Model file for the job. Use its own axes, mm. A direction names the side the tool comes from. Give positions to 0.01 mm unless a question says otherwise; leave off trailing zeros. Loops run counter-clockwise (first coordinate to the right, second up) from the corner with the lowest first, then second, coordinate; pieces in that order, holes last. Notation, with made-up numbers: M -1,-22 L 31,-22 A17 cw 31,0 Z; hole C -36.75,-20 d7. An arc over 180 degrees is marked long. Answer in a Markdown table with one row per item.
```python
from build123d import *

# Parameters (mm, degrees)
SKETCH1_W                 = 71.11
SKETCH1_H                 = 53.65
SKETCH1_R                 = 6.35
SKETCH1_R_2               = 1.5
BOSS_EXTRUDE1_DEPTH       = 6.35
F_8_CLEARANCE_HOLE1_D     = 4.4958
F_6_32_TAPPED_HOLE1_D     = 2.7051
F_6_32_TAPPED_HOLE1_DEPTH = 25.4
F_6_32_TAPPED_HOLE1_TIP   = 0.81269403
CUT_EXTRUDE1_DEPTH        = 7.35
FILLET1_R                 = 3.175


with BuildPart() as part:
    # Sketch1 → Boss-Extrude1 (new body)
    with BuildSketch(Plane.XY):
        with Locations((0, -0.090978152)):
            Rectangle(SKETCH1_W, SKETCH1_H)
        Circle(SKETCH1_R, mode=Mode.SUBTRACT)
        with Locations((-8, 0)):
            Circle(SKETCH1_R_2, mode=Mode.SUBTRACT)
        with Locations((0, 9.5)):
            Circle(SKETCH1_R_2, mode=Mode.SUBTRACT)
        with Locations((8, 0)):
            Circle(SKETCH1_R_2, mode=Mode.SUBTRACT)
        with Locations((0, -9.5)):
            Circle(SKETCH1_R_2, mode=Mode.SUBTRACT)
    extrude(amount=BOSS_EXTRUDE1_DEPTH)

    # #8 Clearance Hole1 (through all)
    with Locations(Plane(origin=(0, 0, 0), x_dir=(-1, 0, 0), z_dir=(0, 0, -1))):
        with Locations((-29.205, -0.090978152), (29.205, -0.090978152)):
            Hole(F_8_CLEARANCE_HOLE1_D / 2)

    # #6-32 Tapped Hole1
    with Locations(Plane(origin=(0, 26.734021848, 0), x_dir=(1, 0, 0), z_dir=(0, 1, 0))):
        with Locations((15.75, -3.175), (-15.75, -3.175)):
            Hole(F_6_32_TAPPED_HOLE1_D / 2, depth=F_6_32_TAPPED_HOLE1_DEPTH)
            with Locations((0, 0, -(F_6_32_TAPPED_HOLE1_DEPTH + F_6_32_TAPPED_HOLE1_TIP / 2))):  # 118° drill point
                Cone(0, F_6_32_TAPPED_HOLE1_D / 2, F_6_32_TAPPED_HOLE1_TIP, mode=Mode.SUBTRACT)

    # Sketch7 → Cut-Extrude1 (cut, through all)
    with BuildSketch(Plane(origin=(0, 0, 0), x_dir=(-1, 0, 0), z_dir=(0, 0, -1))):
        Polygon((-35.555, 26.734021848), (-35.555, 7.684021848), (-20.40455, 26.734021848), align=None)
        Polygon((35.555, 26.734021848), (20.27755, 26.734021848), (35.555, 7.684021848), align=None)
        with BuildLine():
            Line((-35.555, -26.915978152), (35.555, -26.915978152))
            Line((35.555, -26.915978152), (35.555, -7.865978152))
            ThreePointArc((35.555, -7.865978152), (0, -16.669524425), (-35.555, -7.865978152))
            Line((-35.555, -7.865978152), (-35.555, -26.915978152))
        make_face()
    extrude(amount=-CUT_EXTRUDE1_DEPTH, mode=Mode.SUBTRACT)

    # Fillet1
    fillet1_edges = [part.edges().sort_by_distance(p)[0] for p in [
        (35.555, 7.684021848, 3.175),
        (20.40455, 26.734021848, 3.175),
        (-20.27755, 26.734021848, 3.175),
        (-35.555, 7.684021848, 3.175),
        (35.555, -7.865978152, 3.175),
        (-35.555, -7.865978152, 3.175),
    ]]
    fillet(fillet1_edges, radius=FILLET1_R)


solid = part.part
```
Q1. Mould opens along Z. For faces 3 (the face through (31.281, -0.952, 3.219)), 4 (the face through (-8, 5, 0)), 5 (the face through (-14.4, 13.9, 3.1)) say: released by +Z, released by -Z, zero draft, split by the parting line, or undercut.
Reported:
| item | result |
|---|---|
| face 3 | zero draft |
| face 4 | released by -Z |
| face 5 | undercut |
Q2. Drop flat-ended pins along their axis: pin 1 (1 mm diameter, centred on x = -19.5, z = 4.5, fed in from +Y); pin 2 (20.5 mm diameter, centred on x = 0, y = 0, fed in from +Z); pin 3 (1 mm diameter, centred on y = 16.5, z = 1, fed in from -X); pin 4 (3 mm diameter, centred on x = -15.75, z = 3.175, fed in from -Y). Give the stop position or say it passes through.
Reported:
| item | result |
|---|---|
| pin 1 | y = 26.72 |
| pin 2 | z = 6.35 |
| pin 3 | x = -28.89 |
| pin 4 | y = -15.33 |
Q3. Saw through at A-A (x = 0). Give the cut face in (y, z).
Reported:
| item | result |
|---|---|
| outline | M -16.67,0 L -11,0 L -11,6.35 L -16.67,6.35 Z; M -8,0 L -6.35,0 L -6.35,6.35 L -8,6.35 Z; M 6.35,0 L 8,0 L 8,6.35 L 6.35,6.35 Z; M 11,0 L 26.73,0 L 26.73,6.35 L 11,6.35 Z |
Q4. Probe probe 1 along Y at (x, z) = (0, 1.5); probe 2 along X at (y, z) = (-2, 4.5) (3 decimals); probe 3 along X at (y, z) = (15.5, 4.25). List the from-to ranges inside material, lowest first.
Reported:
| item | result |
|---|---|
| probe 1 | -16.67 to -11, -8 to -6.35, 6.35 to 8, 11 to 26.73 |
| probe 2 | -35.555 to -30.392, -28.018 to -6.027, 6.027 to 28.018, 30.392 to 35.555 |
| probe 3 | -29.29 to -16.57, -14.93 to 14.93, 16.57 to 29.34 |
Q5. Saw through at D-D (y = 17.5). Give the cut face in (x, z) (3 decimals), and give its area (3 significant figures).
Reported:
| item | result |
|---|---|
| outline | M -27.683,0 L 27.748,0 L 27.748,6.35 L -27.683,6.35 Z; hole C -15.75,3.175 d2.705; hole C 15.75,3.175 d2.705 |
| area | 340 mm² |
Q6. Saw through at C-C (x = 8). Give the cut face in (y, z).
Reported:
| item | result |
|---|---|
| outline | M -16.25,0 L -1.5,0 L -1.5,6.35 L -16.25,6.35 Z; M 1.5,0 L 26.73,0 L 26.73,6.35 L 1.5,6.35 Z |
Q7. Saw through at B-B (y = -3.5). Give the cut face in (x, z) (3 decimals), and give its area (3 significant figures).
Reported:
| item | result |
|---|---|
| outline | M -35.555,0 L -5.298,0 L -5.298,6.35 L -35.555,6.35 Z; M 5.298,0 L 35.555,0 L 35.555,6.35 L 5.298,6.35 Z |
| area | 384 mm² |
Q8. 3-axis set-ups, long thin cutter, end or side, ignore diameter. For faces 1 (the face through (17.1, 13.9, 3.1)), 2 (the face through (35.555, 0, 3)): which of +Z, -Z, +X, -X, +Y, -Y reach the whole face in a straight line?
Reported:
| item | result |
|---|---|
| face 1 | +Y |
| face 2 | +Z, -Z, +X, +Y, -Y |
